Check sheet for the modelled part. Datum: model origin and axes. Units: mm. A direction names the side the tool comes from. Round coordinates to 2 decimals unless told otherwise and drop trailing zeros. Order: outer loops, then holes, each group sorted by start corner. A loop starts at its lowest first (then second) coordinate and runs counter-clockwise, first axis right, second up.
(1) Mould release check, pull along Y, two halves, no side actions. Record for faces 4 (the cylindrical face through (-6.09, -9.43, 7.4)), 5 (the flat face through (-6, 0, -6)), 6 (the flat face through (37.9, 0, -1)): released by +Y, released by -Y, zero draft, split by the parting line, or undercut.
(2) Sectioned sample at B-B, the plane z = -11. Enter the section's corners in (x, y).
(3) Thickness scan on probe 1 along Z at (x, y) = (38.4, -3); probe 2 along X at (y, z) = (5.25, 17); probe 3 along Z at (x, y) = (-3.5, 0.25). Record the ranges inside material, lowest first.
(4) Tool access check on faces 1 (the flat face through (-6, 0, 6)), 2 (the flat face through (37.9, 0, 16)), 3 (the flat face through (-6, 0, -8)). Record the directions out of +Z, -Z, +X, -X, +Y, -Y that give a thin tool (end or side, any length) a straight path to the whole face; none if there is none.
(5) Sectioned sample at A-A, the plane x = 25. Enter the section's corners in (y, z).
(6) Sectioned sample at D-D, the plane z = 3.9. Enter the section's corners in (x, y), and give its area (3 significant figures).
(7) Sectioned sample at C-C, the plane x = 0. Count the separate pieces of the cut face and the enclosed holes in it, and give its area (3 significant figures).
(8) Depth check by flat-ended pin: pin 1 (1.3 mm diameter, centred on x = 11.4, z = 19.9, fed in from +Y); pin 2 (5 mm diameter, centred on x = -6, y = 0.5, fed in from -Z). Enter the tip coordinate at first touch or a pass-through.
```python
from build123d import *

# Parameters (mm, degrees)
BOSS_EXTRUDE3_DEPTH      = 3.9
BOSS_EXTRUDE3_DEPTH_BACK = 16.1
SKETCH8_R                = 1.089581078
CUT_EXTRUDE2_DEPTH       = 23.9
SKETCH9_R                = 1.096990471
CUT_EXTRUDE3_DEPTH       = 23.9
SKETCH14_W               = 60
SKETCH14_H               = 22
BOSS_EXTRUDE4_DEPTH      = 42
CUT_EXTRUDE4_DEPTH       = 22
CUT_EXTRUDE4_DEPTH_BACK  = 25
FILLET5_R                = 0.25
SKETCH20_R               = 1.1
CUT_EXTRUDE6_DEPTH       = 110
SKETCH23_R               = 1.1
CUT_EXTRUDE7_DEPTH       = 110


with BuildPart() as part:
    # Sketch1 → Boss-Extrude3 (new body, two sides)
    with BuildSketch(Plane(origin=(0, 0, 0), x_dir=(0, 0, -1), z_dir=(1, 0, 0))) as boss_extrude3_sk:
        with BuildLine():
            ThreePointArc((-6, -10), (-7.414213562, -9.414213562), (-8, -8))
            Line((-8, -8), (-8, 8))
            ThreePointArc((-8, 8), (-7.414213562, 9.414213562), (-6, 10))
            Line((-6, 10), (6, 10))
            ThreePointArc((6, 10), (7.414213562, 9.414213562), (8, 8))
            Line((8, 8), (8, -8))
            ThreePointArc((8, -8), (7.414213562, -9.414213562), (6, -10))
            Line((6, -10), (-6, -10))
        make_face()
        with BuildLine():
            ThreePointArc((-6, -7.25), (-5.926776695, -7.426776695), (-5.75, -7.5))
            Line((-5.75, -7.5), (5.75, -7.5))
            ThreePointArc((5.75, -7.5), (5.926776695, -7.426776695), (6, -7.25))
            Line((6, -7.25), (6, 7.25))
            ThreePointArc((6, 7.25), (5.926776695, 7.426776695), (5.75, 7.5))
            Line((5.75, 7.5), (-5.75, 7.5))
            ThreePointArc((-5.75, 7.5), (-5.926776695, 7.426776695), (-6, 7.25))
            Line((-6, 7.25), (-6, -7.25))
        make_face(mode=Mode.SUBTRACT)
    extrude(amount=BOSS_EXTRUDE3_DEPTH)
    extrude(boss_extrude3_sk.sketch, amount=-BOSS_EXTRUDE3_DEPTH_BACK)

    # Sketch8 → Cut-Extrude2 (cut)
    with BuildSketch(Plane.XY.offset(8)):
        with Locations((0, 5.960174238)):
            Circle(SKETCH8_R)
    extrude(amount=-CUT_EXTRUDE2_DEPTH, mode=Mode.SUBTRACT)

    # Sketch9 → Cut-Extrude3 (cut)
    with BuildSketch(Plane.XY.offset(-8)):
        with Locations((0.217674261, -5.978268898)):
            Circle(SKETCH9_R)
    extrude(amount=CUT_EXTRUDE3_DEPTH, mode=Mode.SUBTRACT)

    # Sketch14 → Boss-Extrude4 (add)
    with BuildSketch(Plane(origin=(3.9, 0, 0), x_dir=(0, 0, -1), z_dir=(1, 0, 0))):
        Rectangle(SKETCH14_W, SKETCH14_H)
    extrude(amount=BOSS_EXTRUDE4_DEPTH)

    # Sketch19 → Cut-Extrude4 (cut, two sides)
    with BuildSketch(Plane(origin=(0, 0, 0), x_dir=(1, 0, 0), z_dir=(0, 1, 0))) as cut_extrude4_sk:
        Polygon((11.9, -23.5), (19.2, -23.5), (19.2, -25), (30.6, -25), (30.6, -23.5), (37.9, -23.5), (37.9, 23.5), (11.9, 23.5), align=None)
    extrude(amount=CUT_EXTRUDE4_DEPTH, mode=Mode.SUBTRACT)
    extrude(cut_extrude4_sk.sketch, amount=-CUT_EXTRUDE4_DEPTH_BACK, mode=Mode.SUBTRACT)

    # Fillet5
    fillet5_edges = [part.edges().sort_by_distance(p)[0] for p in [
        (3.9, -11, 0),
        (3.9, 0, 30),
        (3.9, 0, -30),
        (24.9, -11, -30),
        (3.9, 11, 0),
        (24.9, 11, -30),
        (45.9, 0, 30),
        (24.9, 11, 30),
        (45.9, -11, 0),
        (24.9, -11, 30),
        (45.9, 0, -30),
        (45.9, 11, 0),
        (3.9, -9.414213562, 7.414213562),
        (3.9, -10, 0),
        (3.9, 9.414213562, -7.414213562),
        (3.9, 0, 8),
        (3.9, -9.414213562, -7.414213562),
        (3.9, 0, -8),
        (3.9, 10, 0),
        (3.9, 9.414213562, 7.414213562),
    ]]
    fillet(fillet5_edges, radius=FILLET5_R)

    # Sketch20 → Cut-Extrude6 (cut)
    with BuildSketch(Plane(origin=(0, 11, 0), x_dir=(1, 0, 0), z_dir=(0, 1, 0))):
        with Locations((11.4, 5.5)):
            Circle(SKETCH20_R)
        with Locations((11.4, -3.9)):
            Circle(SKETCH20_R)
        with Locations((11.4, -11.9)):
            Circle(SKETCH20_R)
        with Locations((11.4, -19.9)):
            Circle(SKETCH20_R)
        with Locations((38.4, -19.9)):
            Circle(SKETCH20_R)
        with Locations((38.4, -11.9)):
            Circle(SKETCH20_R)
        with Locations((38.4, -3.9)):
            Circle(SKETCH20_R)
        with Locations((38.4, 5.5)):
            Circle(SKETCH20_R)
    extrude(amount=-CUT_EXTRUDE6_DEPTH, mode=Mode.SUBTRACT)

    # Sketch23 → Cut-Extrude7 (cut)
    with BuildSketch(Plane(origin=(0, 11, 0), x_dir=(1, 0, 0), z_dir=(0, 1, 0))):
        with Locations((16.9, -24)):
            Circle(SKETCH23_R)
        with Locations((32.9, -24)):
            Circle(SKETCH23_R)
    extrude(amount=-CUT_EXTRUDE7_DEPTH, mode=Mode.SUBTRACT)


solid = part.part
```
Derived:
1. face 4: released by -Y
1. face 5: undercut
1. face 6: zero draft
2. outline: (3.9, -10.75) arc R0.25 ccw to (4.15, -11) - (11.9, -11) - (11.9, 11) - (4.15, 11) arc R0.25 ccw to (3.9, 10.75) - close; (37.9, -11) - (45.65, -11) arc R0.25 ccw to (45.9, -10.75) - (45.9, 10.75) arc R0.25 ccw to (45.65, 11) - (37.9, 11) - close
3. probe 1: z = -30 to -6.6, -4.4 to 2.8, 5 to 10.8, 13 to 18.8, 21 to 30
3. probe 2: x = 3.9 to 11.9, 37.9 to 45.9
3. probe 3: z = -8 to -6, 6 to 8
4. face 1: -X
4. face 2: +Y, -Y
4. face 3: -Z, -X, +Y, -Y
5. outline: (-11, -29.75) arc R0.25 ccw to (-10.75, -30) - (10.75, -30) arc R0.25 ccw to (11, -29.75) - (11, -23.5) - (-11, -23.5) - close; (-11, 25) - (11, 25) - (11, 29.75) arc R0.25 ccw to (10.75, 30) - (-10.75, 30) arc R0.25 ccw to (-11, 29.75) - close
6. outline: (-16.1, -10) - (3.65, -10) arc R0.25 cw to (3.9, -10.25) - (3.9, -10.75) arc R0.25 ccw to (4.15, -11) - (10.3, -11) - (10.3, 11) - (4.15, 11) arc R0.25 ccw to (3.9, 10.75) - (3.9, 10.25) arc R0.25 cw to (3.65, 10) - (-16.1, 10) - (-16.1, 7.5) - (3.9, 7.5) - (3.9, -7.5) - (-16.1, -7.5) - close; (39.5, -11) - (45.65, -11) arc R0.25 ccw to (45.9, -10.75) - (45.9, 10.75) arc R0.25 ccw to (45.65, 11) - (39.5, 11) - close
6. area: 382 mm2
7. separate pieces: 4
7. enclosed holes: 0
7. area: 119 mm2
8. pin 1: passes through
8. pin 2: stops at z = -8
